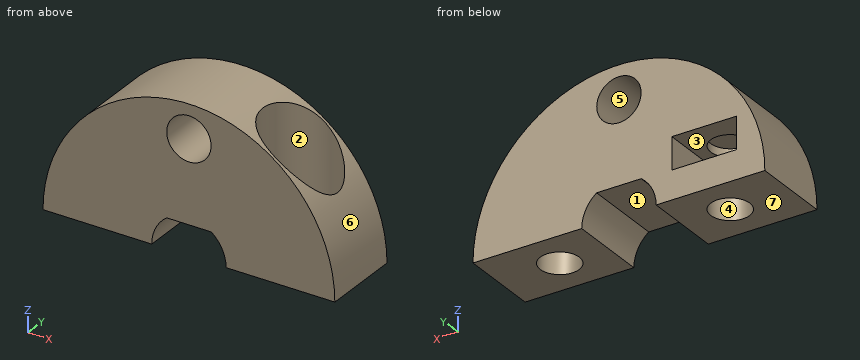
Autodesk Inventor part; units mm, degrees
ref_plane "Work Plane1" through (0, 0, 2.5) normal (0, 0, 1) x (1, 0, 0)
ref_plane "Work Plane2" through (0, 0, -2.5) normal (0, 0, 1) x (1, 0, 0)
ref_plane "Work Plane3" through (0, 5.3975, 0) normal (0, 1, 0) x (1, 0, 0)
sketch "Sketch1" plane through (0, 0, 0) normal (0, 1, 0) x (-1, 0, 0)
  circle A0 centre (0, 0) radius 12.7
  dimension "d75" = 25.4
extrude "Extrusion1" add sketch "Sketch1" along normal blind 3.4925 and the other way blind 3.4925
ref_plane "Work Plane1" through (0, 0, 2.5) normal (0, 0, 1) x (1, 0, 0)
ref_plane "Work Plane2" through (0, 0, -2.5) normal (0, 0, 1) x (1, 0, 0)
sketch "Sketch2" plane through (0, 0, 0) normal (0, 0, 1) x (1, 0, 0)
  circle A0 centre (7.4168, 0) radius 1.7
  circle A1 centre (-7.4168, 0) radius 1.7
  point P0 (0, 0)
  dimension "d5" = 3.4
  dimension "d6" = 7.4168
  dimension "d7" = 3.4
  dimension "d8" = 7.4168
extrude "Screw hole 2" cut sketch "Sketch2" along normal blind 2.5 and the other way blind 6 contours A0
sketch "Sketch3" plane through (0, 0, 2.5) normal (0, 0, 1) x (1, 0, 0)
  circle A0 centre (7.4168, 0) radius 1.7
  circle A1 centre (7.4168, 0) radius 3.25
  point P0 (0, 0)
  dimension "d19" = 6.5
sketch "Sketch4" plane through (0, 0, -2.5) normal (0, 0, 1) x (1, 0, 0)
  circle A0 centre (7.4168, 0) radius 1.7
  circle A1 centre (7.4168, 0) radius 3.45 construction
  line L0 (7.4168, -3.45) -> (4.429, -1.725)
  line L1 (4.429, -1.725) -> (4.429, 6.985)
  line L2 (10.4046, 6.985) -> (10.4046, -1.725)
  line L3 (10.4046, -1.725) -> (7.4168, -3.45)
  line L4 (10.4046, 6.985) -> (4.429, 6.985)
  point P0 (0, 0)
  dimension "d22" = 6.9
sketch "Sketch5" plane through (0, 0, -2.5) normal (0, 0, 1) x (1, 0, 0)
  circle A0 centre (-7.422, 0) radius 3.25
  point P0 (0, 0)
  dimension "d25" = 6.5
extrude "Access Hole 1" cut sketch "Sketch5" against normal through all
extrude "Access Hole 2" cut sketch "Sketch3" along normal through all contours A0 | A1
extrude "Nut well 2" cut sketch "Sketch4" against normal blind 2.794 contours A0 | L0 L1 L4 L2 L3
sketch "Sketch7" plane through (0, 0, 2.5) normal (0, 0, 1) x (1, 0, 0)
  circle A0 centre (-7.422, 0) radius 3.25 construction
  circle A1 centre (-7.422, 0) radius 3.45 construction
  line L0 (-7.422, -3.25) -> (-10.2365, -1.625)
  line L1 (-10.2365, -1.625) -> (-10.2365, 5.3975)
  line L2 (-4.6074, 5.3975) -> (-4.6074, -1.625)
  line L3 (-4.6074, -1.625) -> (-7.422, -3.25)
  line L4 (16.6201, 5.3975) -> (-16.6201, 5.3975)
  line L5 (-10.2365, 5.3975) -> (-4.6074, 5.3975)
  point P0 (0, 0)
  dimension "d48" = 6.9
extrude "Nut Well 1" cut sketch "Sketch7" along normal blind 2.794
sketch "Sketch8" plane through (0, 0, 0) normal (0, 0, 1) x (1, 0, 0)
  circle A0 centre (-7.422, 0) radius 3.25
  circle A1 centre (-7.422, 0) radius 1.7
  point P0 (0, 0)
  dimension "d51" = 3.4
extrude "Screw Hole 1" cut sketch "Sketch8" along normal blind 6 and the other way blind 2.5 contours A1
ref_plane "Work Plane3" through (0, 5.3975, 0) normal (0, 1, 0) x (1, 0, 0)
sketch "Sketch9" plane through (0, 5.3975, 0) normal (0, 1, 0) x (1, 0, 0)
  arc A0 (1.9431, -2.5908) -> (-1.9431, -2.5908) centre (0, 0) ccw
  line L0 (-1.9431, -2.5908) -> (1.9431, -2.5908)
  dimension "d56" = 6.477
  dimension "d57" = 2.5908
extrude "Center shaft" cut sketch "Sketch9" against normal through all
ref_plane "Work Plane4" through (0, 5.3975, 0) normal (0, 1, 0) x (1, 0, 0)
sketch "Sketch10" plane through (0, 5.3975, 0) normal (0, 1, 0) x (1, 0, 0)
  circle A0 centre (0, 9.779) radius 1.9304
  circle A1 centre (0, -9.779) radius 1.9304
  point P0 (0, 0)
  point P1 (0, -8.001)
  dimension "d60" = 3.8608
  dimension "d61" = 9.779
  dimension "d62" = 3.8608
  dimension "d63" = 9.779
extrude "Wheel holes" cut sketch "Sketch10" against normal through all
split "Split1" plane through (0, 0, 0) removes the side toward (0, 0, -1)
properties part number "clamping hub .770 .25 D bore left"
Source: CAD feature listing. Evaluate the final solid. Frame: model axes, mm. Face numbers are marked on the shaded views. A direction names the side the tool comes from. Give positions to 0.01 mm unless a question says otherwise; leave off trailing zeros. Order: outer loops, then holes, each group sorted by start corner. A loop starts at its lowest first (then second) coordinate and runs counter-clockwise, first axis right, second up. Notation, with made-up numbers: (65.25, 61) -> (108.25, 61) arc R25 ccw to (108.25, 73) -> close; hole circle Ø10 at (36.5, 21). An arc over 180 degrees is marked (long way). Use a Markdown table: item, result.
Q1. Section A-A (x = 0). Return the cut outline in (y, z), and give its area (3 significant figures).
A:
| item | result |
|---|---|
| outline | (-3.49, 2.59) -> (3.49, 2.59) -> (3.49, 7.85) -> (-3.49, 7.85) -> close; (-3.49, 11.71) -> (3.49, 11.71) -> (3.49, 12.7) -> (-3.49, 12.7) -> close |
| area | 43.6 mm^2 |
Q2. Section C-C (y = 0). Return the cut outline in (x, z).
A:
| item | result |
|---|---|
| outline | (-12.7, 0) -> (-9.12, 0) -> (-9.12, 2.5) -> (-10.24, 2.5) -> (-10.24, 5.29) -> (-9.12, 5.29) -> (-9.12, 6) -> (-5.72, 6) -> (-5.72, 5.29) -> (-4.61, 5.29) -> (-4.61, 2.5) -> (-5.72, 2.5) -> (-5.72, 0) -> (-3.24, 0) arc R3.24 cw to (-1.94, 2.59) -> (1.94, 2.59) arc R3.24 cw to (3.24, 0) -> (5.72, 0) -> (5.72, 2.5) -> (4.17, 2.5) -> (4.17, 12) arc R12.7 ccw to start; (9.12, 0) -> (12.7, 0) arc R12.7 ccw to (10.67, 6.89) -> (10.67, 2.5) -> (9.12, 2.5) -> close; hole circle Ø3.86 at (0, 9.78) |
Q3. Section B-B (z = 1.75). Return the cut outline in (x, y).
A:
| item | result |
|---|---|
| outline | (-12.58, -3.49) -> (-2.72, -3.49) -> (-2.72, 3.49) -> (-12.58, 3.49) -> close; (2.72, -3.49) -> (12.58, -3.49) -> (12.58, 3.49) -> (2.72, 3.49) -> close; hole circle Ø3.4 at (-7.42, 0); hole circle Ø3.4 at (7.42, 0) |
Q4. First-contact query: P1, Ø1, axis at y = -1, z = 4.5, coming from the -X side; P2, Ø1.5, axis at x = 1, y = -2.5, coming from the -Z side; P3, Ø1.5, axis at y = -1.5, z = 5, coming from the -X side. Flat tips, straight axial feed; report the tip coordinate or a pass-through.
A:
| item | result |
|---|---|
| P1 | x = -12.05 |
| P2 | z = 2.59 |
| P3 | x = -11.97 |
Q5. Material intervals for line 1 (X direction, y = 0, z = 5.45); line 2 (X direction, y = 0, z = 0.55); line 3 (X direction, y = 0, z = 0.95), sorted ascending. Write a range as [from, to].
A:
| item | result |
|---|---|
| line 1 | [-11.47, -9.12], [-5.72, 4.17], [10.67, 11.47] |
| line 2 | [-12.69, -9.12], [-5.72, -3.19], [3.19, 5.72], [9.12, 12.69] |
| line 3 | [-12.66, -9.12], [-5.72, -3.1], [3.1, 5.72], [9.12, 12.66] |
Q6. Pull-direction query (X, two-part tool) for the marked faces 5, 6 and 7; classes: +X half, -X half, draft (parallel to the pull), parting line (faces both ways), or undercut.
A:
| item | result |
|---|---|
| face 5 | undercut |
| face 6 | parting line |
| face 7 | draft |
Q7. Section D-D (x = 4.5). Return the cut outline in (y, z), and give its area (3 significant figures).
A:
| item | result |
|---|---|
| outline | (-3.49, 0) -> (3.49, 0) -> (3.49, 11.88) -> (1.43, 11.88) -> (1.43, 2.5) -> (-1.43, 2.5) -> (-1.43, 11.88) -> (-3.49, 11.88) -> close |
| area | 56.1 mm^2 |
Q8. Access query for the marked faces 1, 2, 3 and 4. Directions: +Z, -Z, +X, -X, +Y, -Y. A direction counts if a zero-diameter tool reaches every point of the face in a straight line with its end or side. Return the directions, or none.
A:
| item | result |
|---|---|
| face 1 | -Z, +Y, -Y |
| face 2 | +Z |
| face 3 | +Y |
| face 4 | -Z |
